from build123d import *
from build123d.topology import SkipClean

# Parameters (mm, degrees)
SKETCH1_R                       = 40
SKETCH1_R_2                     = 30
BOSS_EXTRUDE1_DEPTH             = 5
M4X0_7_TAPPED_HOLE1_D           = 3.3
M4X0_7_TAPPED_HOLE1_CSINK_D     = 4.05
M4X0_7_TAPPED_HOLE1_CSINK_ANGLE = 90
CIRPATTERN1_COUNT               = 6
SKETCH14_R                      = 10
BOSS_EXTRUDE5_DEPTH             = 5
BOSS_EXTRUDE7_START             = 15
SKETCH15_R                      = 2.025
SKETCH15_W                      = 15
SKETCH15_H                      = 15
BOSS_EXTRUDE7_DEPTH             = 15
M4X0_7_TAPPED_HOLE2_D           = 3.3
M4X0_7_TAPPED_HOLE2_DEPTH       = 15
M4X0_7_TAPPED_HOLE2_CSINK_D     = 4.05
M4X0_7_TAPPED_HOLE2_CSINK_ANGLE = 90
M4X0_7_TAPPED_HOLE2_TIP         = 0.991420021
FILLET1_R                       = 7
FILLET2_R                       = 2


with BuildPart() as part:
    # Sketch1 → Boss-Extrude1 (new body)
    with BuildSketch(Plane.XY):
        Circle(SKETCH1_R)
        Circle(SKETCH1_R_2, mode=Mode.SUBTRACT)
    extrude(amount=-BOSS_EXTRUDE1_DEPTH)

    # M4x0.7 Tapped Hole1 (through all)
    with Locations(Plane.XY):
        with Locations((36.25, 0)):
            m4x0_7_tapped_hole1 = CounterSinkHole(M4X0_7_TAPPED_HOLE1_D / 2, M4X0_7_TAPPED_HOLE1_CSINK_D / 2, counter_sink_angle=M4X0_7_TAPPED_HOLE1_CSINK_ANGLE)

    # CirPattern1: M4x0.7 Tapped Hole1 ×6 about axis
    cirpattern1_axis = Axis((0, 0, 0), (0, 0, 1))
    for i in range(1, CIRPATTERN1_COUNT):
        add(m4x0_7_tapped_hole1.rotate(cirpattern1_axis, i * 360 / CIRPATTERN1_COUNT), mode=Mode.SUBTRACT)

    # Sketch14 → Boss-Extrude5 (add)
    with BuildSketch(Plane.XY):
        with BuildLine():
            ThreePointArc((39.906916487, -2.727272727), (0, -40), (-39.906916487, -2.727272727))
            Line((-39.906916487, -2.727272727), (-24.941822804, -221.704545455))
            ThreePointArc((-24.941822804, -221.704545455), (0, -245), (24.941822804, -221.704545455))
            Line((24.941822804, -221.704545455), (39.906916487, -2.727272727))
        make_face()
        with Locations((0, -220)):
            Circle(SKETCH14_R, mode=Mode.SUBTRACT)
    extrude(amount=-BOSS_EXTRUDE5_DEPTH)

    # Sketch15 → Boss-Extrude7 (add)
    # profile 1 of 2: a face of its own
    with SkipClean():  # the faces are left unmerged after this step: merging them gives an invalid solid
        with BuildSketch(Plane.XY.offset(BOSS_EXTRUDE7_START)):
            with BuildLine():
                Line((-39.906916487, -2.727272727), (-31.570605203, -124.708648069))
                Line((-31.570605203, -124.708648069), (-19.477143205, -155))
                Line((-19.477143205, -155), (-26.701678828, -49.28672208))
                Line((-26.701678828, -49.28672208), (-10, -38.284271247))
                Line((-10, -38.284271247), (-10, -28.284271247))
                ThreePointArc((-10, -28.284271247), (0, 30), (10, -28.284271247))
                Line((10, -28.284271247), (10, -38.284271247))
                Line((10, -38.284271247), (26.701678828, -49.28672208))
                Line((26.701678828, -49.28672208), (19.477143205, -155))
                Line((19.477143205, -155), (31.570605203, -124.708648069))
                Line((31.570605203, -124.708648069), (39.906916487, -2.727272727))
                ThreePointArc((39.906916487, -2.727272727), (0, 40), (-39.906916487, -2.727272727))
            make_face()
            with Locations((-18.125, -31.393420887)):
                Circle(SKETCH15_R, mode=Mode.SUBTRACT)
            with Locations((-36.25, 0)):
                Circle(SKETCH15_R, mode=Mode.SUBTRACT)
            with Locations((-18.125, 31.393420887)):
                Circle(SKETCH15_R, mode=Mode.SUBTRACT)
            with Locations((36.25, 0)):
                Circle(SKETCH15_R, mode=Mode.SUBTRACT)
            with Locations((18.125, -31.393420887)):
                Circle(SKETCH15_R, mode=Mode.SUBTRACT)
            with Locations((18.125, 31.393420887)):
                Circle(SKETCH15_R, mode=Mode.SUBTRACT)
        # profile 2 of 2: a face of its own
        with BuildSketch(Plane.XY.offset(BOSS_EXTRUDE7_START)):
            with Locations((0, -177.5)):
                Rectangle(SKETCH15_W, SKETCH15_H)
        extrude(amount=-BOSS_EXTRUDE7_DEPTH)

    # M4x0.7 Tapped Hole2
    with Locations(Plane.XY.offset(15)):
        with Locations((0, -177.5), (-27.564144185, -110), (27.564144185, -110), (-30.981186852, -60), (30.981186852, -60)):
            CounterSinkHole(M4X0_7_TAPPED_HOLE2_D / 2, M4X0_7_TAPPED_HOLE2_CSINK_D / 2, depth=M4X0_7_TAPPED_HOLE2_DEPTH, counter_sink_angle=M4X0_7_TAPPED_HOLE2_CSINK_ANGLE)
            with Locations((0, 0, -(M4X0_7_TAPPED_HOLE2_DEPTH + M4X0_7_TAPPED_HOLE2_TIP / 2))):  # 118° drill point
                Cone(0, M4X0_7_TAPPED_HOLE2_D / 2, M4X0_7_TAPPED_HOLE2_TIP, mode=Mode.SUBTRACT)

    # Fillet1
    # the kernel refuses this fillet: 7 mm, written as the material it adds along each edge
    with BuildSketch(Plane(origin=(-26.701678828, -49.28672208, 15), x_dir=(0.8350839414170254, 0.5501225416099637, 0), z_dir=(0, 0, -1))) as fillet1_piece_1:
        with BuildLine():
            CenterArc((FILLET1_R * 0.583582124754, FILLET1_R), FILLET1_R, 209.465856716, 60.534143284)
            Line((-FILLET1_R * 0.287066858092, FILLET1_R * 0.508095183324), (0, 0))
            Line((0, 0), (FILLET1_R * 0.583582124754, 0))
        make_face()
    extrude(amount=15)
    with BuildSketch(Plane(origin=(26.701678828, -49.28672208, 15), x_dir=(-0.8350839414170222, 0.5501225416099685, 0), z_dir=(0, 0, -1))) as fillet1_piece_2:
        with BuildLine():
            CenterArc((FILLET1_R * 0.583582124754, -FILLET1_R), FILLET1_R, 90, 60.534143284)
            Line((-FILLET1_R * 0.287066858092, -FILLET1_R * 0.508095183324), (0, 0))
            Line((0, 0), (FILLET1_R * 0.583582124754, 0))
        make_face()
    extrude(amount=15)
    # the kernel refuses this fillet: 7 mm, written as the material it takes off along each edge
    with BuildSketch(Plane(origin=(-31.570605203, -124.708648069, 17.748908315), x_dir=(-0.06818181818181737, 0.9976729121658168, 0), z_dir=(0, 0, -1))) as fillet1_2_piece_1:
        with BuildLine():
            CenterArc((FILLET1_R * 0.157080475159, FILLET1_R), FILLET1_R, 252.145796046, 17.854203954)
            Line((-FILLET1_R * 0.149515442954, FILLET1_R * 0.048160232499), (0, 0))
            Line((0, 0), (FILLET1_R * 0.157080475159, 0))
        make_face()
    extrude(amount=17.748908315, mode=Mode.SUBTRACT)
    with BuildSketch(Plane(origin=(-10, -38.284271247, 24.427621741), x_dir=(0, 1, 0), z_dir=(0, 0, -1))) as fillet1_2_piece_2:
        with BuildLine():
            CenterArc((FILLET1_R * 0.538721242354, -FILLET1_R), FILLET1_R, 90, 56.624579759)
            Line((-FILLET1_R * 0.296362699063, -FILLET1_R * 0.44987745839), (0, 0))
            Line((0, 0), (FILLET1_R * 0.538721242354, 0))
        make_face()
    extrude(amount=24.427621741, mode=Mode.SUBTRACT)
    with BuildSketch(Plane(origin=(-10, -28.284271247, 26.447705507), x_dir=(-0.9176733218940842, 0.39733571986907557, 0), z_dir=(0, 0, -1))) as fillet1_2_piece_3:
        with BuildLine():
            CenterArc((4.60428033, -6.983451615), FILLET1_R, 93.940506137, 62.647767091)
            Line((-1.819432923, -4.202101576), (0, 0))
            ThreePointArc((0, 0), (2.061618058, -0.070921648), (4.123236116, 0))
        make_face()
    extrude(amount=26.447705507, mode=Mode.SUBTRACT)
    with BuildSketch(Plane(origin=(10, -28.284271247, 26.447705507), x_dir=(0, -1, 0), z_dir=(0, 0, -1))) as fillet1_2_piece_4:
        with BuildLine():
            CenterArc((4.579082203, -7), FILLET1_R, 90, 62.647767091)
            ThreePointArc((-1.63830899, -3.783783784), (-0.754071591, -1.920071596), (0, 0))
            Line((0, 0), (4.579082203, 0))
        make_face()
    extrude(amount=26.447705507, mode=Mode.SUBTRACT)
    with BuildSketch(Plane(origin=(10, -38.284271247, 24.427621741), x_dir=(0, 1, 0), z_dir=(0, 0, -1))) as fillet1_2_piece_5:
        with BuildLine():
            CenterArc((FILLET1_R * 0.538721242354, FILLET1_R), FILLET1_R, 213.375420241, 56.624579759)
            Line((-FILLET1_R * 0.296362699063, FILLET1_R * 0.44987745839), (0, 0))
            Line((0, 0), (FILLET1_R * 0.538721242354, 0))
        make_face()
    extrude(amount=24.427621741, mode=Mode.SUBTRACT)
    with BuildSketch(Plane(origin=(31.570605203, -124.708648069, 17.748908315), x_dir=(0.06818181818181737, 0.9976729121658168, 0), z_dir=(0, 0, -1))) as fillet1_2_piece_6:
        with BuildLine():
            CenterArc((FILLET1_R * 0.157080475159, -FILLET1_R), FILLET1_R, 90, 17.854203954)
            Line((-FILLET1_R * 0.149515442954, -FILLET1_R * 0.048160232499), (0, 0))
            Line((0, 0), (FILLET1_R * 0.157080475159, 0))
        make_face()
    extrude(amount=17.748908315, mode=Mode.SUBTRACT)

    # Fillet2
    fillet2_edges = [part.edges().sort_by_distance(p)[0] for p in [
        (7.5, -170, 7.5),
        (-7.5, -170, 7.5),
        (-7.5, -185, 7.5),
        (7.5, -185, 7.5),
        (-19.477143205, -155, 7.5),
        (19.477143205, -155, 7.5),
    ]]
    fillet(fillet2_edges, radius=FILLET2_R)


solid = part.part
Verification items for the finished model (mm, model axes). A direction names the side the tool comes from. Give positions to 0.01 mm unless a question says otherwise; leave off trailing zeros. Loops run counter-clockwise (first coordinate to the right, second up) from the corner with the lowest first, then second, coordinate; pieces in that order, holes last.
1. Cross-section at A-A on z = 5.75. Count the separate pieces of the cut face and the enclosed holes in it, and give its area (3 significant figures).
Derived:
separate pieces: 2
enclosed holes: 11
area: 4,760 mm2
2. Cross-section at B-B on y = -88.5. Record the cut outline in (x, z), and give its area (3 significant figures).
Derived:
outline: (-34.05, -5) - (34.05, -5) - (34.05, 15) - (24.02, 15) - (24.02, 0) - (-24.02, 0) - (-24.02, 15) - (-34.05, 15) - close
area: 641 mm2
3. Tool access check on faces 1 (the flat face through (27.632, -134.575, 7.605)), 2 (the flat face through (-27.73, -134.33, 7.6)), 3 (the cylindrical face through (-25.735, -49.824, 7.605)). Record the directions out of +Z, -Z, +X, -X, +Y, -Y that give a thin tool (end or side, any length) a straight path to the whole face; none if there is none.
Derived:
face 1: +Z, +X, -Y
face 2: +Z, -X, -Y
face 3: +Z
4. Material ranges on probe 1 along X at (y, z) = (0, 8.5) (3 decimals); probe 2 along Y at (x, z) = (0, -2.4); probe 3 along Y at (x, z) = (-1.5, 5.5), recorded low to high.
Derived:
probe 1: x = -40 to -38.275, -34.225 to -30, 30 to 34.225, 38.275 to 40
probe 2: y = -245 to -230, -210 to -30, 30 to 40
probe 3: y = -185 to -178.19, -176.81 to -170, 29.96 to 39.97
5. Go/stop test with flat-tipped pins: P1, Ø3, axis at x = -18.13, y = -31.39, coming from the -Z side; P2, Ø10, axis at x = 8.5, z = 9, coming from the -Y side; P3, Ø8, axis at y = -72.5, z = 11, coming from the -X side; P4, Ø3, axis at x = -27.56, y = -110, coming from the +Z side. Record where each tip stops, or that it passes through.
Derived:
P1: passes through
P2: stops at y = -185
P3: stops at x = -35.41
P4: stops at z = -0.09
6. Release check for a two-part mould opening along Y. For faces 4 (the cylindrical face through (25.69, -49.73, 7.6)), 5 (the flat face through (-11, -33, 15)), 6 (the cylindrical face through (-10.815, -37.79, 7.605)) record: +Y half, -Y half, draft (parallel to the pull), parting line (faces both ways), or undercut.
Derived:
face 4: undercut
face 5: draft
face 6: -Y half
